Work out the finished part from the listing and answer in its coordinate system (mm). A direction names the side the tool comes from. Coordinates: 2 decimals unless noted, no trailing zeros. Write each question's results on one line, items separated by ' | '.
```python
from build123d import *

# Parameters (mm, degrees)
F0_R          = 1.049364
F1_DEPTH      = 5.08
F1_DEPTH_BACK = 5.08


with BuildPart() as f1:
    # F0 (on Front) → F1 (new body, two sides)
    with BuildSketch(Plane.XZ) as f1_sk:
        with BuildLine():
            ThreePointArc((-37.025139, 22.682322), (-36.964615, 23.310248), (-36.944413, 23.940761))
            ThreePointArc((-36.944413, 23.940761), (-36.945103, 24.057295), (-36.947171, 24.173813))
            ThreePointArc((-36.947171, 24.173813), (-36.997563, 24.962594), (-37.111039, 25.744795))
            ThreePointArc((-37.111039, 25.744795), (-37.275689, 26.473733), (-37.495132, 27.188089))
            ThreePointArc((-37.495132, 27.188089), (-37.785454, 27.923227), (-38.133787, 28.632719))
            ThreePointArc((-38.133787, 28.632719), (-38.514452, 29.275801), (-38.942779, 29.88817))
            ThreePointArc((-38.942779, 29.88817), (-39.444941, 30.498537), (-39.994428, 31.066674))
            ThreePointArc((-39.994428, 31.066674), (-40.554276, 31.561679), (-41.150044, 32.012812))
            ThreePointArc((-41.150044, 32.012812), (-41.81546, 32.439352), (-42.512935, 32.811163))
            ThreePointArc((-42.512935, 32.811163), (-43.366856, 33.17471), (-44.251205, 33.456268))
            ThreePointArc((-44.251205, 33.456268), (-45.022377, 33.629499), (-45.804956, 33.740337))
            ThreePointArc((-45.804956, 33.740337), (-46.550793, 33.7871), (-47.298029, 33.777179))
            ThreePointArc((-47.298029, 33.777179), (-48.085122, 33.705072), (-48.863899, 33.570085))
            ThreePointArc((-48.863899, 33.570085), (-49.588023, 33.385412), (-50.296062, 33.146369))
            ThreePointArc((-50.296062, 33.146369), (-51.022921, 32.835901), (-51.722546, 32.468151))
            ThreePointArc((-51.722546, 32.468151), (-52.354895, 32.069911), (-52.955229, 31.624873))
            ThreePointArc((-52.955229, 31.624873), (-53.551528, 31.106083), (-54.104308, 30.541151))
            ThreePointArc((-54.104308, 30.541151), (-54.583698, 29.967875), (-55.018244, 29.359903))
            ThreePointArc((-55.018244, 29.359903), (-55.426287, 28.682987), (-55.778739, 27.975532))
            ThreePointArc((-55.778739, 27.975532), (-56.058788, 27.282688), (-56.2855, 26.570605))
            ThreePointArc((-56.2855, 26.570605), (-56.465808, 25.801057), (-56.58383, 25.019529))
            ThreePointArc((-56.58383, 25.019529), (-56.637441, 24.274153), (-56.634385, 23.526858))
            ThreePointArc((-56.634385, 23.526858), (-56.569511, 22.739135), (-56.441684, 21.959151))
            ThreePointArc((-56.441684, 21.959151), (-56.26367, 21.233361), (-56.031141, 20.523157))
            ThreePointArc((-56.031141, 20.523157), (-55.727363, 19.793476), (-55.366055, 19.090503))
            ThreePointArc((-55.366055, 19.090503), (-54.97364, 18.454523), (-54.534136, 17.850126))
            ThreePointArc((-54.534136, 17.850126), (-54.020845, 17.249087), (-53.461014, 16.69114))
            ThreePointArc((-53.461014, 16.69114), (-52.892167, 16.206504), (-52.288212, 15.766392))
            ThreePointArc((-52.288212, 15.766392), (-51.615072, 15.352148), (-50.910885, 14.993212))
            ThreePointArc((-50.910885, 14.993212), (-50.220642, 14.706811), (-49.510672, 14.473567))
            ThreePointArc((-49.510672, 14.473567), (-48.742813, 14.286198), (-47.962402, 14.161002))
            ThreePointArc((-47.962402, 14.161002), (-47.21755, 14.100547), (-46.470258, 14.096738))
            ThreePointArc((-46.470258, 14.096738), (-45.681973, 14.154373), (-44.900848, 14.27503))
            ThreePointArc((-44.900848, 14.27503), (-44.173453, 14.446369), (-43.461143, 14.672365))
            ThreePointArc((-43.461143, 14.672365), (-42.728702, 14.969428), (-42.02244, 15.324263))
            ThreePointArc((-42.02244, 15.324263), (-41.382882, 15.710819), (-40.774473, 16.144753))
            ThreePointArc((-40.774473, 16.144753), (-40.168744, 16.652501), (-39.605679, 17.207183))
            ThreePointArc((-39.605679, 17.207183), (-39.115838, 17.771555), (-38.670197, 18.371442))
            ThreePointArc((-38.670197, 18.371442), (-38.249787, 19.040748), (-37.884398, 19.741608))
            ThreePointArc((-37.884398, 19.741608), (-37.591668, 20.429191), (-37.351913, 21.136988))
            ThreePointArc((-37.351913, 21.136988), (-37.157498, 21.903094), (-37.025139, 22.682322))
        make_face()
        with Locations((-46.793749, 23.940761)):
            Circle(F0_R, mode=Mode.SUBTRACT)
        with BuildLine():
            ThreePointArc((-37.111039, 25.744795), (-36.997563, 24.962594), (-36.947171, 24.173813))
            Line((-36.947171, 24.173813), (-35.07041, 25.163614))
            Line((-35.07041, 25.163614), (-37.111039, 25.744795))
        make_face()
        with BuildLine():
            Line((-35.261809, 21.502234), (-37.025139, 22.682322))
            ThreePointArc((-37.025139, 22.682322), (-37.157498, 21.903094), (-37.351913, 21.136988))
            Line((-37.351913, 21.136988), (-35.261809, 21.502234))
        make_face()
        with BuildLine():
            ThreePointArc((-38.133787, 28.632719), (-37.785454, 27.923227), (-37.495132, 27.188089))
            Line((-37.495132, 27.188089), (-36.013299, 28.706677))
            Line((-36.013299, 28.706677), (-38.133787, 28.632719))
        make_face()
        with BuildLine():
            Line((-36.568978, 18.076794), (-37.884398, 19.741608))
            ThreePointArc((-37.884398, 19.741608), (-38.249787, 19.040748), (-38.670197, 18.371442))
            Line((-38.670197, 18.371442), (-36.568978, 18.076794))
        make_face()
        with BuildLine():
            ThreePointArc((-39.994428, 31.066674), (-39.444941, 30.498537), (-38.942779, 29.88817))
            Line((-38.942779, 29.88817), (-37.999248, 31.788615))
            Line((-37.999248, 31.788615), (-39.994428, 31.066674))
        make_face()
        with BuildLine():
            Line((-38.865442, 15.21872), (-39.605679, 17.207183))
            ThreePointArc((-39.605679, 17.207183), (-40.168744, 16.652501), (-40.774473, 16.144753))
            Line((-40.774473, 16.144753), (-38.865442, 15.21872))
        make_face()
        with BuildLine():
            ThreePointArc((-42.512935, 32.811163), (-41.81546, 32.439352), (-41.150044, 32.012812))
            Line((-41.150044, 32.012812), (-40.836107, 34.111235))
            Line((-40.836107, 34.111235), (-42.512935, 32.811163))
        make_face()
        with BuildLine():
            Line((-41.929007, 13.204544), (-42.02244, 15.324263))
            ThreePointArc((-42.02244, 15.324263), (-42.728702, 14.969428), (-43.461143, 14.672365))
            Line((-43.461143, 14.672365), (-41.929007, 13.204544))
        make_face()
        with BuildLine():
            ThreePointArc((-45.804956, 33.740337), (-45.022377, 33.629499), (-44.251205, 33.456268))
            Line((-44.251205, 33.456268), (-44.673904, 35.535514))
            Line((-44.673904, 35.535514), (-45.804956, 33.740337))
        make_face()
        with BuildLine():
            Line((-45.463259, 12.229149), (-44.900848, 14.27503))
            ThreePointArc((-44.900848, 14.27503), (-45.681973, 14.154373), (-46.470258, 14.096738))
            Line((-46.470258, 14.096738), (-45.463259, 12.229149))
        make_face()
        with BuildLine():
            ThreePointArc((-48.863899, 33.570085), (-48.085122, 33.705072), (-47.298029, 33.777179))
            Line((-47.298029, 33.777179), (-48.339167, 35.625954))
            Line((-48.339167, 35.625954), (-48.863899, 33.570085))
        make_face()
        with BuildLine():
            Line((-49.126242, 12.386907), (-47.962402, 14.161002))
            ThreePointArc((-47.962402, 14.161002), (-48.742813, 14.286198), (-49.510672, 14.473567))
            Line((-49.510672, 14.473567), (-49.126242, 12.386907))
        make_face()
        with BuildLine():
            ThreePointArc((-51.722546, 32.468151), (-51.022921, 32.835901), (-50.296062, 33.146369))
            Line((-50.296062, 33.146369), (-51.854904, 34.585796))
            Line((-51.854904, 34.585796), (-51.722546, 32.468151))
        make_face()
        with BuildLine():
            Line((-52.563546, 13.662555), (-50.910885, 14.993212))
            ThreePointArc((-50.910885, 14.993212), (-51.615072, 15.352148), (-52.288212, 15.766392))
            Line((-52.288212, 15.766392), (-52.563546, 13.662555))
        make_face()
        with BuildLine():
            ThreePointArc((-54.104308, 30.541151), (-53.551528, 31.106083), (-52.955229, 31.624873))
            Line((-52.955229, 31.624873), (-54.88095, 32.51568))
            Line((-54.88095, 32.51568), (-54.104308, 30.541151))
        make_face()
        with BuildLine():
            Line((-55.442594, 15.932668), (-53.461014, 16.69114))
            ThreePointArc((-53.461014, 16.69114), (-54.020845, 17.249087), (-54.534136, 17.850126))
            Line((-54.534136, 17.850126), (-55.442594, 15.932668))
        make_face()
        with BuildLine():
            ThreePointArc((-55.778739, 27.975532), (-55.426287, 28.682987), (-55.018244, 29.359903))
            Line((-55.018244, 29.359903), (-57.124521, 29.6159))
            Line((-57.124521, 29.6159), (-55.778739, 27.975532))
        make_face()
        with BuildLine():
            Line((-57.484826, 18.977603), (-55.366055, 19.090503))
            ThreePointArc((-55.366055, 19.090503), (-55.727363, 19.793476), (-56.031141, 20.523157))
            Line((-56.031141, 20.523157), (-57.484826, 18.977603))
        make_face()
        with BuildLine():
            ThreePointArc((-56.58383, 25.019529), (-56.465808, 25.801057), (-56.2855, 26.570605))
            Line((-56.2855, 26.570605), (-58.368541, 26.167024))
            Line((-58.368541, 26.167024), (-56.58383, 25.019529))
        make_face()
        with BuildLine():
            Line((-58.492645, 22.502746), (-56.441684, 21.959151))
            ThreePointArc((-56.441684, 21.959151), (-56.569511, 22.739135), (-56.634385, 23.526858))
            Line((-56.634385, 23.526858), (-58.492645, 22.502746))
        make_face()
    extrude(amount=F1_DEPTH)
    extrude(f1_sk.sketch, amount=-F1_DEPTH_BACK)


solid = f1.part
```
1) Given pin 1 Ø5 at (x, y) = (-45.5, 0) entering from -Z; pin 2 Ø4 at (x, y) = (-39.5, -3) entering from -Z, each flat-ended and moving along its own axis, determine where each tip first touches the part or whether it passes through.
Check result:
pin 1: z = 12.23 | pin 2: z = 15.22
2) Straight lines are drawn through the part: probe 1 along Z at (x, y) = (-43.5, -0.25); probe 2 along X at (y, z) = (-0.75, 28.5); probe 3 along X at (y, z) = (4, 21.75). For each, find the intervals that lie inside material, in ascending order. Write a range as [from, to].
Check result:
probe 1: [14.66, 33.22] | probe 2: [-56.21, -36.21] | probe 3: [-56.4, -35.63]
3) For a pull along X with two mould halves and no side action, classify faces 1 (the face through (-46.54, -0.071, 33.787)), 2 (the face through (-37.27, -0.07, 26.46)), 3 (the face through (-56.461, -0.071, 28.807)), 4 (the face through (-56.44, -0.071, 19.033)) as released by +X, released by -X, zero draft, split by the parting line, or undercut.
Check result:
face 1: undercut | face 2: released by +X | face 3: released by -X | face 4: undercut
4) Which of the six approach directions +Z, -Z, +X, -X, +Y, -Y give full straight-line access (tool end or side, diameter ignored) to faces 5 (the face through (-54.577, -0.071, 29.976)), 6 (the face through (-44.46, -0.07, 34.48)), 7 (the face through (-37.634, -0.071, 18.226)), 8 (the face through (-57.49, -0.07, 25.6))?
Check result:
face 5: +Y, -Y | face 6: +Z, +Y, -Y | face 7: -Z, +Y, -Y | face 8: -X, +Y, -Y
